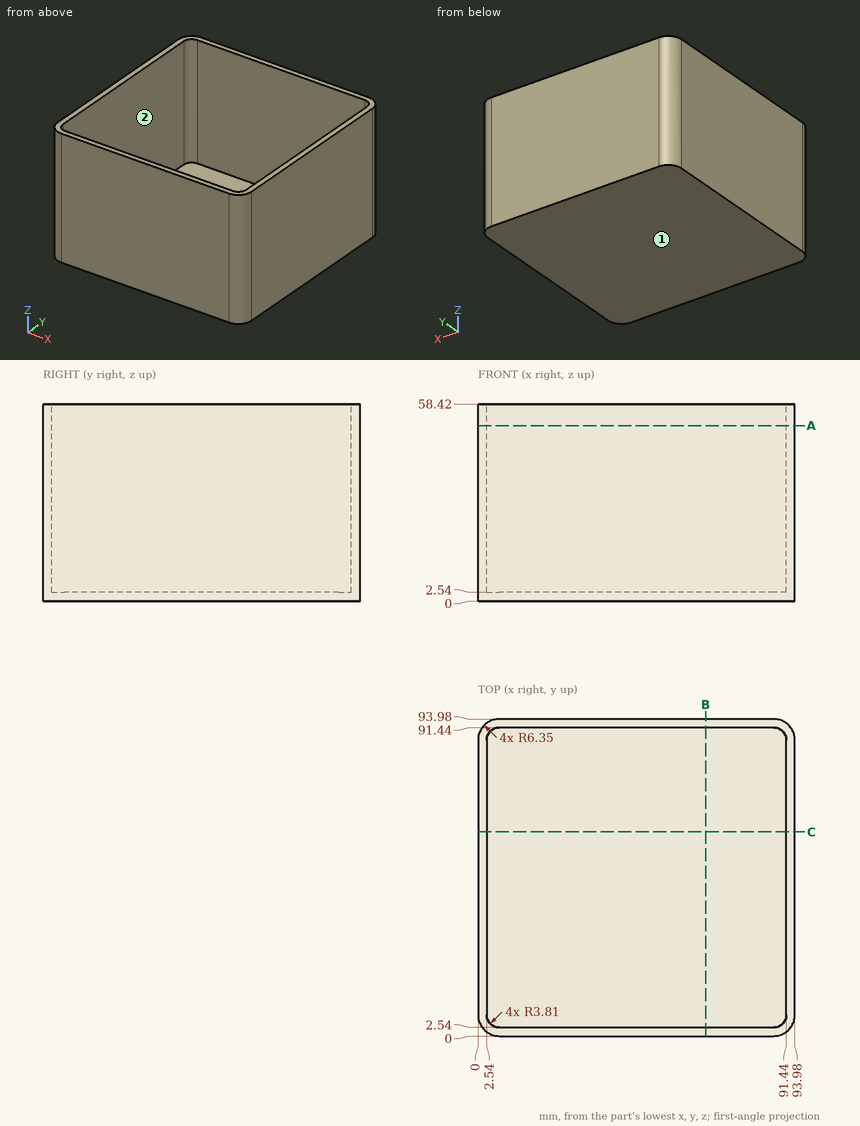
Answer from the drawing. Dimensions are ordinates in mm from the lowest x, y and z of the part. A direction names the side the tool comes from. Give positions to 0.01 mm unless a question says otherwise; leave off trailing zeros. Order: outer loops, then holes, each group sorted by start corner. A loop starts at its lowest first (then second) coordinate and runs counter-clockwise, first axis right, second up. Notation, with made-up numbers: (87, 15) -> (119, 15) arc R18 cw to (119, 48) -> close; hole circle Ø3 at (26.25, 70). An arc over 180 degrees is marked (long way). One line per item, written item: value. Start each with the question number.
(1) A tool of negligible diameter and unlimited length cuts with its end or side. For the marked faces 1 and 2, from which of +Z, -Z, +X, -X, +Y, -Y can it reach the whole face along a straight path? Write none if from no direction.
(2) Flat-ended cylindrical pins translate along their axes: P1, Ø1.5, axis at x = 51, z = 38.5, coming from the -Y side; P2, Ø5, axis at x = 75, y = 20.5, coming from the +Z side. Find the tip coordinate at first contact, or state that the pin passes through.
(3) Straight lines are drawn through the part: L1, parallel to X at y = 10.5, z = 21; L2, parallel to Z at x = 10, y = 63. For each, find the intervals that lie inside material, in ascending order.
(4) The part is cut by section A-A (z = 52). Determine the outline of the cut face in (x, y).
(5) The part is cut by section B-B (x = 67.5). Determine the outline of the cut face in (y, z).
Taken from the geometry:
1. face 1: -Z, +X, -X, +Y, -Y
1. face 2: +Z
2. P1: y = 0
2. P2: z = 2.54
3. L1: 0 to 2.54, 91.44 to 93.98
3. L2: 0 to 2.54
4. outline: (0, 6.35) arc R6.35 ccw to (6.35, 0) -> (87.63, 0) arc R6.35 ccw to (93.98, 6.35) -> (93.98, 87.63) arc R6.35 ccw to (87.63, 93.98) -> (6.35, 93.98) arc R6.35 ccw to (0, 87.63) -> close; hole (2.54, 6.35) arc R3.81 ccw to (6.35, 2.54) -> (87.63, 2.54) arc R3.81 ccw to (91.44, 6.35) -> (91.44, 87.63) arc R3.81 ccw to (87.63, 91.44) -> (6.35, 91.44) arc R3.81 ccw to (2.54, 87.63) -> close
5. outline: (0, 0) -> (93.98, 0) -> (93.98, 58.42) -> (91.44, 58.42) -> (91.44, 2.54) -> (2.54, 2.54) -> (2.54, 58.42) -> (0, 58.42) -> close
